Read the model definition and answer for the solid it produces. Units are mm, in the model's axes. Face numbers are marked on the shaded views. A direction names the side the tool comes from. Round coordinates to 2 decimals unless told otherwise and drop trailing zeros. Write each loop counter-clockwise with the first axis right and the second up, starting at its lowest first coordinate (ties: lowest second). Pieces come first, ordered by that corner, then holes. Notation, with made-up numbers: (-12.75, 59) -> (45.25, 59) arc R25 cw to (45.25, 83) -> close; hole circle Ø7 at (67.25, 73). An arc over 180 degrees is marked (long way). Return JSON: item names as keys, results as strings. Group by question number.
(1) Straight lines are drawn through the part: line 1 (Y direction, x = 0, z = 11); line 2 (Y direction, x = 0, z = -19.6) (3 decimals); line 3 (Y direction, x = -23, z = 8.5). For each, find the intervals that lie inside material, in ascending order.
(2) Given pin 1 (12 mm diameter, centred on x = -30.5, z = 0.5, fed in from -Y); pin 2 (5 mm diameter, centred on x = 23, y = 22, fed in from -Z); pin 3 (8.5 mm diameter, centred on x = -14.5, y = 11, fed in from -Z), each flat-ended and moving along its own axis, determine where each tip first touches the part or whether it passes through.
(3) For the marked faces 4, 5 and 6, determine the directions among +Z, -Z, +X, -X, +Y, -Y from which every point of the face is accessible in a straight line to the end or side of a thin tool.
(4) A cutting plane is placed at D-D on y = -19. Give the vertices of the cut face in (x, z), then the cut area to 3 significant figures.
(5) The mould has two halves that part along X. Classify the marked faces 1, 2 and 3: released by +X, released by -X, zero draft, split by the parting line, or undercut.
(6) A cutting plane is placed at C-C on z = -16. Give the vertices of the cut face in (x, y), then the cut area to 3 significant figures.
(7) A cutting plane is placed at A-A on x = -12. Give the vertices of the cut face in (y, z), then the cut area to 3 significant figures.
(8) A cutting plane is placed at B-B on y = -27.5. Give the vertices of the cut face in (x, z) (3 decimals).
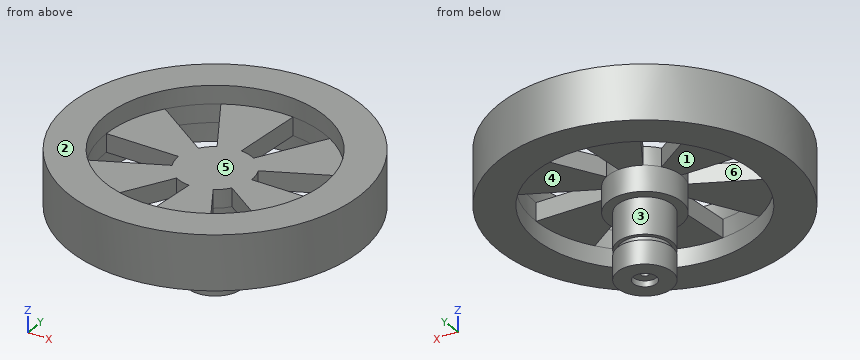
```python
from build123d import *

# Parameters (mm, degrees)
SKETCH1_R           = 40
BOSS_EXTRUDE1_DEPTH = 15
SKETCH2_R           = 7.5
SKETCH2_R_2         = 1
BOSS_EXTRUDE2_DEPTH = 20
SKETCH4_R           = 3.175
CUT_EXTRUDE1_DEPTH  = 1.6
SKETCH5_W           = 2
SKETCH5_H           = 2.576429586
SKETCH5_W_2         = 1.5
SKETCH5_H_2         = 1
SKETCH5_4_W         = 1.5
SKETCH5_4_H         = 1
CUT_EXTRUDE2_START  = -5
SKETCH6_R           = 30
SKETCH6_R_2         = 10.076429586
CUT_EXTRUDE2_DEPTH  = 5
SKETCH7_R           = 30
CUT_EXTRUDE3_DEPTH  = 5
CUT_EXTRUDE4_START  = -5
CUT_EXTRUDE4_DEPTH  = 5


with BuildPart() as part:
    # Sketch1 → Boss-Extrude1 (new body)
    with BuildSketch(Plane.XY):
        Circle(SKETCH1_R)
    extrude(amount=BOSS_EXTRUDE1_DEPTH)

    # Sketch2 → Boss-Extrude2 (add)
    with BuildSketch(Plane.XY):
        Circle(SKETCH2_R)
        Circle(SKETCH2_R_2, mode=Mode.SUBTRACT)
    extrude(amount=-BOSS_EXTRUDE2_DEPTH)

    # Sketch4 → Cut-Extrude1 (cut)
    with BuildSketch(Plane(origin=(0, 0, -20), x_dir=(-1, 0, 0), z_dir=(0, 0, -1))):
        Circle(SKETCH4_R)
    extrude(amount=-CUT_EXTRUDE1_DEPTH, mode=Mode.SUBTRACT)

    # Sketch5 → Revolve2 (revolve)
    with BuildSketch(Plane(origin=(0, 0, 0), x_dir=(0, 0, -1), z_dir=(1, 0, 0)), mode=Mode.PRIVATE) as revolve2_sk:
        with Locations((1, 8.788214793)):
            Rectangle(SKETCH5_W, SKETCH5_H)
        with Locations((12.75, 7)):
            Rectangle(SKETCH5_W_2, SKETCH5_H_2)
    revolve(revolve2_sk.sketch.rotate(Axis((0, 0, -21.75), (0, 0, 1)), 270), axis=Axis((0, 0, -21.75), (0, 0, 1)))

    # Sketch5_4 → Cut-Revolve1 (revolve, cut)
    with BuildSketch(Plane(origin=(0, 0, 0), x_dir=(0, 0, -1), z_dir=(1, 0, 0)), mode=Mode.PRIVATE) as cut_revolve1_sk:
        with Locations((12.75, 7)):
            Rectangle(SKETCH5_4_W, SKETCH5_4_H)
    revolve(cut_revolve1_sk.sketch.rotate(Axis((0, 0, -21.75), (0, 0, 1)), 90), axis=Axis((0, 0, -21.75), (0, 0, 1)), mode=Mode.SUBTRACT)

    # Sketch6 → Cut-Extrude2 (cut)
    with BuildSketch(Plane(origin=(0, 0, 0), x_dir=(-1, 0, 0), z_dir=(0, 0, -1)).offset(CUT_EXTRUDE2_START)):
        Circle(SKETCH6_R)
        Circle(SKETCH6_R_2, mode=Mode.SUBTRACT)
    extrude(amount=CUT_EXTRUDE2_DEPTH, mode=Mode.SUBTRACT)

    # Sketch7 → Cut-Extrude3 (cut)
    with BuildSketch(Plane.XY.offset(15)):
        with Locations(Location((0, 0, 0), (0, 0, 180))):
            Circle(SKETCH7_R)
    extrude(amount=-CUT_EXTRUDE3_DEPTH, mode=Mode.SUBTRACT)

    # Sketch8 → Cut-Extrude4 (cut)
    with BuildSketch(Plane(origin=(0, 0, 5), x_dir=(-1, 0, 0), z_dir=(0, 0, -1)).offset(CUT_EXTRUDE4_START)):
        with BuildLine():
            Line((-10.076429586, 0), (-30, 0))
            ThreePointArc((-30, 0), (-29.266323118, 6.59411337), (-27.101177924, 12.865696838))
            Line((-27.101177924, 12.865696838), (-9.102770368, 4.321342942))
            ThreePointArc((-9.102770368, 4.321342942), (-9.830001471, 2.214837302), (-10.076429586, 0))
        make_face()
        with BuildLine():
            Line((-2.408568663, 29.903156974), (-0.808992418, 10.043901854))
            ThreePointArc((-0.808992418, 10.043901854), (-2.996895367, 9.620449644), (-5.038214793, 8.726444001))
            Line((-5.038214793, 8.726444001), (-15, 25.980762114))
            ThreePointArc((-15, 25.980762114), (-8.922491865, 28.642435981), (-2.408568663, 29.903156974))
        make_face()
        with BuildLine():
            Line((24.692609261, 17.037460136), (8.29377795, 5.722558913))
            ThreePointArc((8.29377795, 5.722558913), (6.833106104, 7.405612342), (5.038214793, 8.726444001))
            Line((5.038214793, 8.726444001), (15, 25.980762114))
            ThreePointArc((15, 25.980762114), (20.343831253, 22.048322611), (24.692609261, 17.037460136))
        make_face()
        with BuildLine():
            Line((27.101177924, -12.865696838), (9.102770368, -4.321342942))
            ThreePointArc((9.102770368, -4.321342942), (9.830001471, -2.214837302), (10.076429586, 0))
            Line((10.076429586, 0), (30, 0))
            ThreePointArc((30, 0), (29.266323118, -6.59411337), (27.101177924, -12.865696838))
        make_face()
        with BuildLine():
            Line((2.408568663, -29.903156974), (0.808992418, -10.043901854))
            ThreePointArc((0.808992418, -10.043901854), (2.996895367, -9.620449644), (5.038214793, -8.726444001))
            Line((5.038214793, -8.726444001), (15, -25.980762114))
            ThreePointArc((15, -25.980762114), (8.922491865, -28.642435981), (2.408568663, -29.903156974))
        make_face()
        with BuildLine():
            Line((-24.692609261, -17.037460136), (-8.29377795, -5.722558913))
            ThreePointArc((-8.29377795, -5.722558913), (-6.833106104, -7.405612342), (-5.038214793, -8.726444001))
            Line((-5.038214793, -8.726444001), (-15, -25.980762114))
            ThreePointArc((-15, -25.980762114), (-20.343831253, -22.048322611), (-24.692609261, -17.037460136))
        make_face()
    extrude(amount=CUT_EXTRUDE4_DEPTH, mode=Mode.SUBTRACT)


solid = part.part
```
Checks:
{
 "1": {"line 1": "y = -40 to -30, 30 to 40", "line 2": "y = -7.5 to -3.175, 3.175 to 7.5", "line 3": "y = -32.73 to -10.92, 0 to 15.87, 19.26 to 32.73"},
 "2": {"pin 1": "stops at y = -31.62", "pin 2": "stops at z = 0", "pin 3": "stops at z = 5"},
 "3": {"face 4": "-Z", "face 5": "+Z", "face 6": "+Z, -Z"},
 "4": {"outline": "(-35.2, 0) -> (-23.22, 0) -> (-23.22, 5) -> (-10.97, 5) -> (-10.97, 10) -> (-23.22, 10) -> (-23.22, 15) -> (-35.2, 15) -> close; (-1.53, 5) -> (10.97, 5) -> (10.97, 10) -> (-1.53, 10) -> close; (23.22, 0) -> (35.2, 0) -> (35.2, 15) -> (23.22, 15) -> close", "area": "483 mm^2"},
 "5": {"face 1": "undercut", "face 2": "zero draft", "face 3": "split by the parting line"},
 "6": {"outline": "circle Ø15 at (0, 0); hole circle Ø2 at (0, 0)", "area": "174 mm^2"},
 "7": {"outline": "(-38.16, 0) -> (-27.5, 0) -> (-27.5, 15) -> (-38.16, 15) -> close; (-20.78, 5) -> (-5.7, 5) -> (-5.7, 10) -> (-20.78, 10) -> close; (0, 5) -> (8.28, 5) -> (8.28, 10) -> (0, 10) -> close; (20.78, 5) -> (27.5, 5) -> (27.5, 0) -> (38.16, 0) -> (38.16, 15) -> (27.5, 15) -> (27.5, 10) -> (20.78, 10) -> close", "area": "470 mm^2"},
 "8": {"outline": "(-29.047, 0) -> (-11.99, 0) -> (-11.99, 15) -> (-29.047, 15) -> close; (-2.215, 5) -> (11.99, 5) -> (11.99, 0) -> (29.047, 0) -> (29.047, 15) -> (11.99, 15) -> (11.99, 10) -> (-2.215, 10) -> close"}
}
